from build123d import *

# Parameters (mm, degrees)
SKETCH1_R                            = 2.0193
BOSS_EXTRUDE1_DEPTH                  = 25.4
F_10_32_TAPPED_HOLE1_D               = 4.0386
F_10_32_TAPPED_HOLE1_DEPTH           = 12.02944
F_10_32_TAPPED_HOLE1_TIP             = 1.213317848
F_10_32_TAPPED_HOLE1_ON_FACE_2_D     = 4.0386
F_10_32_TAPPED_HOLE1_ON_FACE_2_DEPTH = 12.02944
F_10_32_TAPPED_HOLE1_ON_FACE_2_TIP   = 1.213317848


with BuildPart() as part:
    # Sketch1 → Boss-Extrude1 (new body)
    with BuildSketch(Plane.XY):
        with BuildLine():
            ThreePointArc((0.893039571, 6.816751782), (0, 6.874999966), (-0.893039571, 6.816751782))
            Line((-0.893039571, 6.816751782), (-5.456960429, 4.181770846))
            ThreePointArc((-5.456960429, 4.181770846), (-5.953924622, 3.437499983), (-6.35, 2.634980936))
            Line((-6.35, 2.634980936), (-6.35, -2.634980936))
            ThreePointArc((-6.35, -2.634980936), (-5.953924622, -3.437499983), (-5.456960429, -4.181770846))
            Line((-5.456960429, -4.181770846), (-0.893039571, -6.816751782))
            ThreePointArc((-0.893039571, -6.816751782), (0, -6.874999966), (0.893039571, -6.816751782))
            Line((0.893039571, -6.816751782), (5.456960429, -4.181770846))
            ThreePointArc((5.456960429, -4.181770846), (5.953924622, -3.437499983), (6.35, -2.634980936))
            Line((6.35, -2.634980936), (6.35, 2.634980936))
            ThreePointArc((6.35, 2.634980936), (5.953924622, 3.437499983), (5.456960429, 4.181770846))
            Line((5.456960429, 4.181770846), (0.893039571, 6.816751782))
        make_face()
        Circle(SKETCH1_R, mode=Mode.SUBTRACT)
    extrude(amount=BOSS_EXTRUDE1_DEPTH)

    # #10-32 Tapped Hole1
    with Locations(Plane.XY.offset(25.4)):
        with Locations((0, 0)):
            Hole(F_10_32_TAPPED_HOLE1_D / 2, depth=F_10_32_TAPPED_HOLE1_DEPTH)
            with Locations((0, 0, -(F_10_32_TAPPED_HOLE1_DEPTH + F_10_32_TAPPED_HOLE1_TIP / 2))):  # 118° drill point
                Cone(0, F_10_32_TAPPED_HOLE1_D / 2, F_10_32_TAPPED_HOLE1_TIP, mode=Mode.SUBTRACT)

    # #10-32 Tapped Hole1 on face 2
    with Locations(Plane.XY):
        with Locations((0, 0)):
            Hole(F_10_32_TAPPED_HOLE1_ON_FACE_2_D / 2, depth=F_10_32_TAPPED_HOLE1_ON_FACE_2_DEPTH)
            with Locations((0, 0, -(F_10_32_TAPPED_HOLE1_ON_FACE_2_DEPTH + F_10_32_TAPPED_HOLE1_ON_FACE_2_TIP / 2))):  # 118° drill point
                Cone(0, F_10_32_TAPPED_HOLE1_ON_FACE_2_D / 2, F_10_32_TAPPED_HOLE1_ON_FACE_2_TIP, mode=Mode.SUBTRACT)


solid = part.part
Here's how the part is built. I have some questions about the finished solid (model axes, mm). Give positions to 0.01 mm unless a question says otherwise; leave off trailing zeros. Order: outer loops, then holes, each group sorted by start corner. A loop starts at its lowest first (then second) coordinate and runs counter-clockwise, first axis right, second up. Notation, with made-up numbers: M 53.25,-11.75 L 102.25,-11.75 A18 cw 102.25,-7.75 Z; hole C -22,50.25 d2. An arc over 180 degrees is marked long. Answer as a JSON object with one key per item and string values. Group by question number.
1) We'd pull the mould along Y, two halves only. Please class faces 1 (the cylindrical face through (-0.013, -6.875, 12.522)), 2 (the cylindrical face through (1.926, 0.607, 12.522)), 3 (the flat face through (-2, 2, 25.4)), 4 (the cylindrical face through (5.96, 3.43, 12.52)): pulls with the +Y half, pulls with the -Y half, needs draft (parallel to the pull), parting line crosses it, or undercut.
2) Suppose I cut it at B-B, the plane z = 23. Write out the boundary of the cut face in (x, y) (3 decimals).
3) Please list where these lines run through material, in increasing order: L1, parallel to X at y = 0, z = 6.5; L2, parallel to Y at x = 0, z = 6.25 (3 decimals); L3, parallel to Y at x = -0.75, z = 10.75. Write a range as [from, to].
4) Suppose I cut it at C-C, the plane x = 0. Write out the boundary of the cut face in (y, z) (3 decimals).
5) I'm going to push flat-ended pins straight in: pin 1 Ø2 at (x, z) = (3.5, 5) entering from -Y; pin 2 Ø1 at (x, z) = (1, 11.5) entering from -Y; pin 3 Ø6 at (x, z) = (-5, 7) entering from +Y. Where does each tip first touch, or does it pass through?
6) Suppose I cut it at A-A, the plane y = -1. Write out the boundary of the cut face in (x, z).
7) Suppose I cut it at D-D, the plane x = 4.75. Write out the boundary of the cut face in (y, z).
Results found:
{
 "1": {"face 1": "pulls with the -Y half", "face 2": "undercut", "face 3": "needs draft", "face 4": "pulls with the +Y half"},
 "2": {"outline": "M -6.35,-2.635 A6.875 ccw -5.457,-4.182 L -0.893,-6.817 A6.875 ccw 0.893,-6.817 L 5.457,-4.182 A6.875 ccw 6.35,-2.635 L 6.35,2.635 A6.875 ccw 5.457,4.182 L 0.893,6.817 A6.875 ccw -0.893,6.817 L -5.457,4.182 A6.875 ccw -6.35,2.635 Z; hole C 0,0 d4.039"},
 "3": {"L1": "[-6.35, -2.02], [2.02, 6.35]", "L2": "[-6.875, -2.019], [2.019, 6.875]", "L3": "[-6.83, -1.87], [1.87, 6.83]"},
 "4": {"outline": "M -6.875,0 L -2.019,0 L -2.019,25.4 L -6.875,25.4 Z; M 2.019,0 L 6.875,0 L 6.875,25.4 L 2.019,25.4 Z"},
 "5": {"pin 1": "y = -5.89", "pin 2": "y = -6.86", "pin 3": "y = 6.18"},
 "6": {"outline": "M -6.35,0 L -1.75,0 L -1.75,25.4 L -6.35,25.4 Z; M 1.75,0 L 6.35,0 L 6.35,25.4 L 1.75,25.4 Z"},
 "7": {"outline": "M -4.59,0 L 4.59,0 L 4.59,25.4 L -4.59,25.4 Z"}
}
